```python
from build123d import *

# Parameters (mm, degrees)
ESQUISSE1_R             = 14.625
ESQUISSE1_R_2           = 11.625
BOSS_EXTRU_1_DEPTH      = 46.6
BOSS_EXTRU_3_START      = -5
BOSS_EXTRU_3_DEPTH      = 5
ESQUISSE3_W             = 10
ESQUISSE3_H             = 10
BOSS_EXTRU_4_DEPTH      = 5
CONG_1_R                = 5
BOSS_EXTRU_6_START      = -2.5
BOSS_EXTRU_6_DEPTH      = 5
CONG_2_R                = 5
ESQUISSE5_R             = 1.5
ENL_V_MAT_EXTRU_1_DEPTH = 62.452832522
CONG_3_R                = 1.5
CONG_4_R                = 1.5


with BuildPart() as part:
    # Esquisse1 → Boss.-Extru.1 (new body)
    with BuildSketch(Plane.XY):
        Circle(ESQUISSE1_R)
        Circle(ESQUISSE1_R_2, mode=Mode.SUBTRACT)
    extrude(amount=BOSS_EXTRU_1_DEPTH)

    # Esquisse2 → Boss.-Extru.3 (add)
    with BuildSketch(Plane.XY.offset(46.6).offset(BOSS_EXTRU_3_START)):
        with BuildLine():
            Line((-30, 5), (-13.743748579, 5))
            ThreePointArc((-13.743748579, 5), (-14.625, 0), (-13.743748579, -5))
            Line((-13.743748579, -5), (-30, -5))
            Line((-30, -5), (-30, 5))
        make_face()
        with BuildLine():
            Line((30, 5), (30, -5))
            Line((30, -5), (13.743748579, -5))
            ThreePointArc((13.743748579, -5), (14.625, 0), (13.743748579, 5))
            Line((13.743748579, 5), (30, 5))
        make_face()
    extrude(amount=BOSS_EXTRU_3_DEPTH)

    # Esquisse3 → Boss.-Extru.4 (add)
    with BuildSketch(Plane.XY.offset(46.6)):
        with Locations((-25, 0)):
            Rectangle(ESQUISSE3_W, ESQUISSE3_H)
        with Locations((25, 0)):
            Rectangle(ESQUISSE3_W, ESQUISSE3_H)
    extrude(amount=BOSS_EXTRU_4_DEPTH)

    # Congé1
    cong_1_edges = [part.edges().sort_by_distance(p)[0] for p in [
        (30, 0, 41.6),
        (-30, 0, 41.6),
    ]]
    fillet(cong_1_edges, radius=CONG_1_R)

    # Esquisse4 → Boss.-Extru.6 (add)
    with BuildSketch(Plane(origin=(0, 5, 0), x_dir=(1, 0, 0), z_dir=(0, 1, 0)).offset(BOSS_EXTRU_6_START)):
        Polygon((-18.743748579, -41.6), (-13.743748579, -41.6), (-13.743748579, -27.457864376), align=None)
        Polygon((13.743748579, -27.457864376), (13.743748579, -41.6), (18.743748579, -41.6), align=None)
    extrude(amount=-BOSS_EXTRU_6_DEPTH)

    # Congé2
    cong_2_edges = [part.edges().sort_by_distance(p)[0] for p in [
        (20, 0, 46.6),
        (-20, 0, 46.6),
    ]]
    fillet(cong_2_edges, radius=CONG_2_R - 0.0001)  # a hair under: the kernel refuses the full size

    # Esquisse5 → Enlèv. mat.-Extru.1 (cut, through all)
    with BuildSketch(Plane.XY.offset(51.6)):
        with Locations((-25, 0)):
            Circle(ESQUISSE5_R)
        with Locations(Location((25, 0, 0), (0, 0, 270))):
            Circle(ESQUISSE5_R)
    extrude(amount=-ENL_V_MAT_EXTRU_1_DEPTH, mode=Mode.SUBTRACT)

    # Congé3
    cong_3_edges = [part.edges().sort_by_distance(p)[0] for p in [
        (-30, 0, 51.6),
        (-20, 0, 51.6),
        (20, 0, 51.6),
        (30, 0, 51.6),
    ]]
    fillet(cong_3_edges, radius=CONG_3_R)

    # Congé4
    cong_4_edges = [part.edges().sort_by_distance(p)[0] for p in [
        (-11.625, 0, 0),
        (-11.625, 0, 46.6),
    ]]
    fillet(cong_4_edges, radius=CONG_4_R)


solid = part.part
```
Verification items for the finished model (mm, model axes). A direction names the side the tool comes from. Round coordinates to 2 decimals unless told otherwise and drop trailing zeros. Order: outer loops, then holes, each group sorted by start corner. A loop starts at its lowest first (then second) coordinate and runs counter-clockwise, first axis right, second up. Notation, with made-up numbers: (0, 35.25) - (40, 35.25) arc R26 ccw to (40, 51.25) - close; hole circle Ø5 at (3.5, 35.25). An arc over 180 degrees is marked (long way). Use CSV: the item, a comma, the result in double quotes.
(1) Access from +Z, -Z, +X, -X, +Y, -Y to the whole of each face (thin tool, end or side, straight path). Record for faces 4 (the face through (-22, -5, 47)), 5 (the face through (16, 2.5, 38)), 6 (the face through (16, -2.5, 38)), 7 (the face through (-16, 2.5, 38)), 8 (the face through (21, 0, 41.6)).
Entries:
face 4,"+Z, -Z, -X, -Y"
face 5,"-Z, +X, +Y"
face 6,"-Z, +X, -Y"
face 7,"-Z, -X, +Y"
face 8,"-Z, +X"
(2) Mould release check, pull along X, two halves, no side actions. Record for faces 1 (the face through (23, 0, 51.6)), 2 (the face through (-28.57, 0.07, 43.1)), 3 (the face through (-18.064, 0.07, 47.649)): released by +X, released by -X, zero draft, split by the parting line, or undercut.
Entries:
face 1,"zero draft"
face 2,"released by -X"
face 3,"undercut"
(3) Thickness scan on probe 1 along Y at (x, z) = (0, 34) (3 decimals); probe 2 along X at (y, z) = (0, 48.75); probe 3 along X at (y, z) = (0, 49.5). Record the ranges inside material, lowest first. Write a range as from..to.
Entries:
probe 1,"-14.625..-11.625, 11.625..14.625"
probe 2,"-30..-26.5, -23.5..-19.11, 19.11..23.5, 26.5..30"
probe 3,"-30..-26.5, -23.5..-19.54, 19.54..23.5, 26.5..30"
(4) Section check B-B on z = 48. Record the boundary of the cut face in (x, y).
Entries:
outline,"(-30, -5) - (-18.47, -5) - (-18.47, 5) - (-30, 5) - close; (18.47, -5) - (30, -5) - (30, 5) - (18.47, 5) - close; hole circle Ø3 at (-25, 0); hole circle Ø3 at (25, 0)"
(5) Gauge pin test, flat ends, axial feed: pin 1 Ø10 at (x, z) = (6.5, 16) entering from +Y; pin 2 Ø1.5 at (y, z) = (11, 14.5) entering from -X; pin 3 Ø3 at (x, z) = (-18.5, 44) entering from +Y. Record the tip position at first contact, or that the pin passes through.
Entries:
pin 1,"y = 14.55"
pin 2,"x = -10.43"
pin 3,"y = 5"
(6) Section check A-A on x = 0. Record the boundary of the cut face in (y, z) (3 decimals), and give its area (3 significant figures).
Entries:
outline,"(-14.625, 0) - (-13.125, 0) arc R1.5 ccw to (-11.625, 1.5) - (-11.625, 45.1) arc R1.5 ccw to (-13.125, 46.6) - (-14.625, 46.6) - close; (11.625, 1.5) arc R1.5 ccw to (13.125, 0) - (14.625, 0) - (14.625, 46.6) - (13.125, 46.6) arc R1.5 ccw to (11.625, 45.1) - close"
area,"278 mm^2"
(7) Section check C-C on z = 8. Record the boundary of the cut face in (x, y) (3 decimals).
Entries:
outline,"circle Ø29.25 at (0, 0); hole circle Ø23.25 at (0, 0)"
(8) Section check D-D on y = 0. State how many separate pieces and enclosed holes the cut face has, and give its area (3 significant figures).
Entries:
separate pieces,"4"
enclosed holes,"0"
area,"518 mm^2"
